```python
from build123d import *

# Parameters (mm, degrees)
F1_DEPTH = 4.45


# Not quite as in the source:
# - ends of sketch curves that miss each other by under 0.0002 mm in the source are joined


with BuildPart() as f1:
    # F0 (on Front) → F1 (new body)
    with BuildSketch(Plane.XZ):
        with BuildLine():
            Line((2.225, 93.35), (2.225, 88.9))
            Line((2.225, 88.9), (-2.225, 88.9))
            Line((-2.225, 88.9), (-2.225, 93.35))
            Line((-2.225, 93.35), (-32.1837038577, 93.35))
            Line((-32.1837038577, 93.35), (-32.1837038577, 88.9))
            Line((-32.1837038577, 88.9), (-36.6337038577, 88.9))
            Line((-36.6337038577, 88.9), (-36.6337038577, 93.35))
            Line((-36.6337038577, 93.35), (-52.1105349839, 93.35))
            Line((-52.1105349839, 93.35), (-52.1105349839, 88.9))
            Line((-52.1105349839, 88.9), (-56.5605349839, 88.9))
            Line((-56.5605349839, 88.9), (-56.5605349839, 93.35))
            Line((-56.5605349839, 93.35), (-86.2080463052, 93.35))
            Line((-86.2080463052, 93.35), (-86.2080463052, 88.9))
            Line((-86.2080463052, 88.9), (-90.6580463052, 88.9))
            Line((-90.6580463052, 88.9), (-90.6580463052, 93.35))
            Line((-90.6580463052, 93.35), (-95.6580463052, 93.35))
            Line((-95.6580463052, 93.35), (-95.6580463052, 80.85))
            ThreePointArc((-95.6580463052, 80.85), (0, 68.6427723395), (95.6580463052, 80.85))
            Line((95.6580463052, 80.85), (95.6580463052, 93.35))
            Line((95.6580463052, 93.35), (90.6580463052, 93.35))
            Line((90.6580463052, 93.35), (90.6580454826, 88.9))
            Line((90.6580454826, 88.9), (86.2080454826, 88.9))
            Line((86.2080454826, 88.9), (86.2080454826, 93.35))
            Line((86.2080454826, 93.35), (56.5605341613, 93.35))
            Line((56.5605341613, 93.35), (56.5605341613, 88.9))
            Line((56.5605341613, 88.9), (52.1105341613, 88.9))
            Line((52.1105341613, 88.9), (52.1105341613, 93.35))
            Line((52.1105341613, 93.35), (36.6337030351, 93.35))
            Line((36.6337030351, 93.35), (36.6337030351, 88.9))
            Line((36.6337030351, 88.9), (32.1837030351, 88.9))
            Line((32.1837030351, 88.9), (32.1837030351, 93.35))
            Line((32.1837030351, 93.35), (2.225, 93.35))
        make_face()
    extrude(amount=F1_DEPTH)


solid = f1.part
```
Can you work these out from the model? Positions are in its coordinate system, mm. A direction names the side the tool comes from. Coordinates: 2 decimals unless noted, no trailing zeros. Order: outer loops, then holes, each group sorted by start corner. A loop starts at its lowest first (then second) coordinate and runs counter-clockwise, first axis right, second up.
1. For faces 4 (the face through (-32.184, -2, 91)), 5 (the face through (-71, -2, 93.35)), which set-ups out of +Z, -Z, +X, -X, +Y, -Y let a thin tool reach every point of the face, with its end or its side?
2. If we section it at D-D (x = -72): Please give me the cut outline in (y, z).
3. I need wall thicknesses on line 1 (Z direction, x = -0.5, y = -4.2); line 2 (Z direction, x = 3, y = -3.5). Which ranges of each line are inside material? Lowest first, please.
4. If we section it at A-A (z = 91): Give the number of separate pieces and of enclosed holes in the cut face, then the cut area to 3 significant figures.
5. I'm going to push a flat-ended pin straight in: pin 1 (1.3 mm diameter, centred on x = -35, y = -1, fed in from +Z). Where does the tip first touch, or does it pass through?
6. Thinking about a two-plate mould opening in X: for faces 1 (the face through (-1, 0, 81)), 2 (the face through (-95.658, -2, 87)), 3 (the face through (-36.634, -2, 91)), which applies, +X half, -X half, draft (parallel to the pull), parting line (faces both ways), or undercut?
Entries:
1. face 4: +Z, +Y, -Y
1. face 5: +Z, +X, -X, +Y, -Y
2. outline: (-4.45, 75.51) - (0, 75.51) - (0, 93.35) - (-4.45, 93.35) - close
3. line 1: z = 68.64 to 88.9
3. line 2: z = 68.65 to 93.35
4. separate pieces: 8
4. enclosed holes: 0
4. area: 713 mm2
5. pin 1: stops at z = 88.9
6. face 1: draft
6. face 2: -X half
6. face 3: undercut
